Could you check a few things on this model? Use its own coordinates, in mm. Face numbers are marked on the shaded views. A direction names the side the tool comes from. Give positions to 0.01 mm unless a question says otherwise; leave off trailing zeros. Write each loop counter-clockwise with the first axis right and the second up, starting at its lowest first coordinate (ties: lowest second). Pieces come first, ordered by that corner, then holes. Notation, with made-up numbers: (-33, -8) - (17, -8) arc R28 cw to (17, 28) - close; hole circle Ø8 at (-32.5, -12.5). An arc over 180 degrees is marked (long way). Answer as CSV lines item,"result". Start each with the question number.
Q1. Imagine slicing it at C-C on x = 15.25. List the corners of the cut face in (y, z) for me.
Q2. If I drill on line 1 along X through (y, z) = (3, 16.5); line 2 along X through (y, z) = (-2.25, 14.5); line 3 along Z through (x, y) = (4.25, 0.25), over which ranges is the centre line in solid material (lowest first)?
Q3. On a 3-axis mill with a long thin cutter (end or side, diameter ignored), from which of +Z, -Z, +X, -X, +Y, -Y can I reach the whole of each face in a straight line? I mean the marked faces 4, 5, 6 and 7. Say none if no direction works.
Q4. Imagine slicing it at A-A on z = 2. List the corners of the cut face in (x, y) for me.
Q5. Will these pins go through, and if not, where does the flat tip stop? pin 1 Ø4 at (y, z) = (2, 2.5) entering from -X; pin 2 Ø3 at (x, z) = (20.5, 17.5) entering from -Y; pin 3 Ø4 at (x, y) = (16, 1.5) entering from +Z.
Q6. We'd pull the mould along Z, two halves only. Please class the marked faces 1, 2 and 3: pulls with the +Z half, pulls with the -Z half, needs draft (parallel to the pull), parting line crosses it, or undercut.
Q7. Imagine slicing it at D-D on z = 10.75. List the corners of the cut face in (x, y) for me, and give its area (3 significant figures).
```python
from build123d import *

# Parameters (mm, degrees)
SKETCH1_W                     = 3.7
SKETCH1_H                     = 0.65
BOSS_EXTRUDE1_DEPTH           = 6.5
SKETCH2_W                     = 10.6
SKETCH2_H                     = 8.2
BOSS_EXTRUDE2_DEPTH           = 16
SKETCH6_W                     = 4.6
SKETCH6_H                     = 10
CUT_EXTRUDE2_DEPTH            = 0.2
FILLET3_R                     = 0.5
FILLET3_OF_MIRROR2_R          = 0.5
FILLET1_R                     = 1.5
FILLET2_R                     = 0.5
SKETCH3_R                     = 3.75
BOSS_EXTRUDE3_DEPTH           = 9
BOSS_EXTRUDE3_TAPER           = 3
BOSS_EXTRUDE3_OTHER_WAY_DEPTH = 8.7
SKETCH5_W                     = 1
SKETCH5_H                     = 2.895184441
CUT_EXTRUDE1_DEPTH            = 3.35
SKETCH4_R                     = 2.25
BOSS_EXTRUDE4_DEPTH           = 15


with BuildPart() as part:
    # Sketch1 → Boss-Extrude1 (new body)
    with BuildSketch(Plane.XY):
        Polygon((1, 1.8), (0, 1), (0, 0), (6.8, 0), (6.8, 1), (5.8, 1.8), align=None)
        with Locations((3.4, 0.525)):
            Rectangle(SKETCH1_W, SKETCH1_H, mode=Mode.SUBTRACT)
    extrude(amount=BOSS_EXTRUDE1_DEPTH)

    # Sketch2 → Boss-Extrude2 (add)
    with BuildSketch(Plane.XY.offset(6.5)):
        with Locations((3.4, 0.9)):
            Rectangle(SKETCH2_W, SKETCH2_H)
    extrude(amount=BOSS_EXTRUDE2_DEPTH)

    # Sketch6 → Cut-Extrude2 (cut)
    with BuildSketch(Plane(origin=(0, 5, 0), x_dir=(1, 0, 0), z_dir=(0, 1, 0))):
        with Locations((3.4, -14.5)):
            Rectangle(SKETCH6_W, SKETCH6_H)
    cut_extrude2 = extrude(amount=-CUT_EXTRUDE2_DEPTH, mode=Mode.SUBTRACT)

    # Fillet3
    fillet3_edges = [part.edges().sort_by_distance(p)[0] for p in [
        (5.7, 4.9, 9.5),
        (5.7, 4.9, 19.5),
        (1.1, 4.9, 19.5),
        (1.1, 4.9, 9.5),
    ]]
    fillet(fillet3_edges, radius=FILLET3_R)

    # Mirror2: Cut-Extrude2 across plane
    add(cut_extrude2.mirror(Plane.ZX.offset(0.9)), mode=Mode.SUBTRACT)

    # Fillet3 of Mirror2
    fillet3_of_mirror2_edges = [part.edges().sort_by_distance(p)[0] for p in [
        (5.7, -3.1, 9.5),
        (5.7, -3.1, 19.5),
        (1.1, -3.1, 19.5),
        (1.1, -3.1, 9.5),
    ]]
    fillet(fillet3_of_mirror2_edges, radius=FILLET3_OF_MIRROR2_R)

    # Fillet1
    fillet1_edges = [part.edges().sort_by_distance(p)[0] for p in [
        (8.7, 0.9, 22.5),
        (-1.9, 0.9, 22.5),
    ]]
    fillet(fillet1_edges, radius=FILLET1_R)

    # Fillet2
    fillet2_edges = [part.edges().sort_by_distance(p)[0] for p in [
        (3.4, 5, 22.5),
        (3.4, -3.2, 22.5),
        (8.7, -3.2, 13.75),
        (-1.9, -3.2, 13.75),
        (8.260660172, -3.2, 22.060660172),
        (-1.460660172, -3.2, 22.060660172),
        (-1.9, 5, 13.75),
        (8.7, 5, 13.75),
        (8.260660172, 5, 22.060660172),
        (-1.460660172, 5, 22.060660172),
        (8.7, 0.9, 6.5),
        (3.4, 5, 6.5),
        (-1.9, 0.9, 6.5),
        (3.4, -3.2, 6.5),
    ]]
    fillet(fillet2_edges, radius=FILLET2_R)

    # Sketch3 → Boss-Extrude3 (add)
    with BuildSketch(Plane(origin=(8.7, 0, 0), x_dir=(0, 0, -1), z_dir=(1, 0, 0))):
        with Locations((-17.75, 0.9)):
            Circle(SKETCH3_R)
    extrude(amount=BOSS_EXTRUDE3_DEPTH, taper=BOSS_EXTRUDE3_TAPER)

    # Sketch3 → Boss-Extrude3 other way (add)
    with BuildSketch(Plane(origin=(8.7, 0, 0), x_dir=(0, 0, -1), z_dir=(1, 0, 0))):
        with Locations((-17.75, 0.9)):
            Circle(SKETCH3_R)
    extrude(amount=-BOSS_EXTRUDE3_OTHER_WAY_DEPTH)

    # Sketch5 → Cut-Extrude1 (cut)
    with BuildSketch(Plane(origin=(0, 5, 0), x_dir=(1, 0, 0), z_dir=(0, 1, 0))):
        with Locations((11.2, -15.55240778)):
            Rectangle(SKETCH5_W, SKETCH5_H)
        with Locations((13.2, -15.55240778)):
            Rectangle(SKETCH5_W, SKETCH5_H)
        with Locations((15.2, -15.55240778)):
            Rectangle(SKETCH5_W, SKETCH5_H)
        with Locations((11.2, -19.94759222)):
            Rectangle(SKETCH5_W, SKETCH5_H)
        with Locations((13.2, -19.94759222)):
            Rectangle(SKETCH5_W, SKETCH5_H)
        with Locations((15.2, -19.94759222)):
            Rectangle(SKETCH5_W, SKETCH5_H)
    cut_extrude1 = extrude(amount=-CUT_EXTRUDE1_DEPTH, mode=Mode.SUBTRACT)

    # Mirror1: Cut-Extrude1 across plane
    add(cut_extrude1.mirror(Plane.ZX.offset(0.9)), mode=Mode.SUBTRACT)

    # Sketch4 → Boss-Extrude4 (add)
    with BuildSketch(Plane(origin=(8.7, 0, 0), x_dir=(0, 0, -1), z_dir=(1, 0, 0))):
        with Locations((-17.75, 0.9)):
            Circle(SKETCH4_R)
    extrude(amount=BOSS_EXTRUDE4_DEPTH)


solid = part.part
```
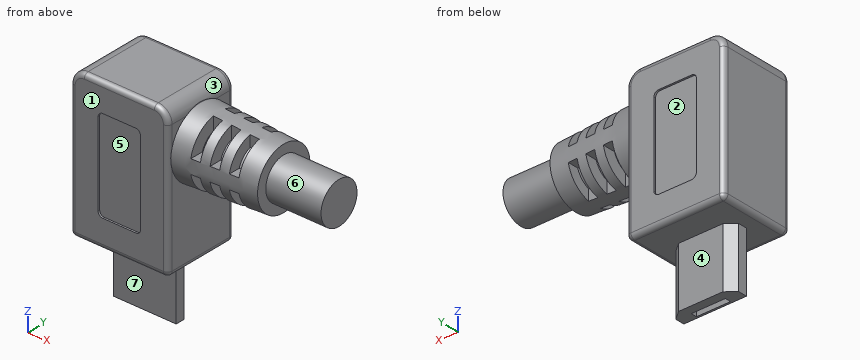
Conclusion:
1,outline,"(-2.42, 17) - (-1.22, 17) arc R2.25 ccw to (0.15, 15.63) - (0.15, 14.43) arc R3.41 ccw to (1.65, 14.43) - (1.65, 15.63) arc R2.25 ccw to (3.02, 17) - (4.22, 17) arc R3.41 ccw to (4.22, 18.5) - (3.02, 18.5) arc R2.25 ccw to (1.65, 19.87) - (1.65, 21.07) arc R3.41 ccw to (0.15, 21.07) - (0.15, 19.87) arc R2.25 ccw to (-1.22, 18.5) - (-2.42, 18.5) arc R3.41 ccw to start"
2,line 1,"-1.9 to 10.7, 11.7 to 12.7, 13.7 to 14.7, 15.7 to 17.7"
2,line 2,"-1.9 to 8.7"
2,line 3,"6.5 to 22.5"
3,face 4,"-Z, +X, -X, +Y"
3,face 5,"-Y"
3,face 6,"+X"
3,face 7,"-Z, +X, -X, -Y"
4,outline,"(0, 0) - (6.8, 0) - (6.8, 1) - (5.8, 1.8) - (1, 1.8) - (0, 1) - close; hole (1.55, 0.2) - (5.25, 0.2) - (5.25, 0.85) - (1.55, 0.85) - close"
5,pin 1,"x = 0"
5,pin 2,"y = -1.35"
5,pin 3,"z = 21.22"
6,face 1,"needs draft"
6,face 2,"undercut"
6,face 3,"pulls with the +Z half"
7,outline,"(-1.9, -2.7) arc R0.5 ccw to (-1.4, -3.2) - (1.1, -3.2) - (1.1, -3) - (5.7, -3) - (5.7, -3.2) - (8.2, -3.2) arc R0.5 ccw to (8.7, -2.7) - (8.7, 4.5) arc R0.5 ccw to (8.2, 5) - (5.7, 5) - (5.7, 4.8) - (1.1, 4.8) - (1.1, 5) - (-1.4, 5) arc R0.5 ccw to (-1.9, 4.5) - close"
7,area,"84.9 mm^2"
